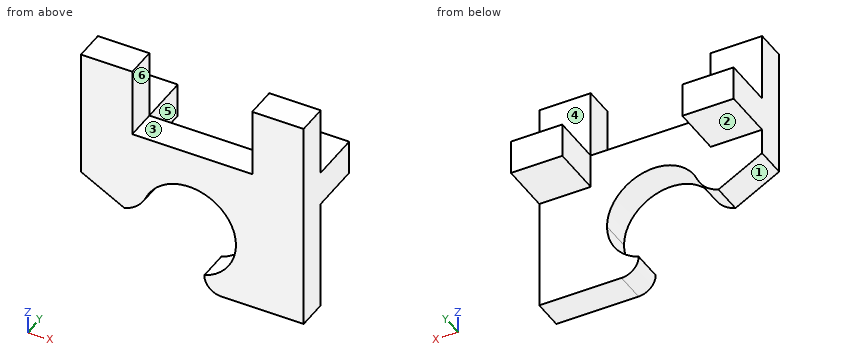
```python
from build123d import *

# Parameters (mm, degrees)
BOSS_EXTRUDE1_DEPTH = 1.8
FILLET1_R           = 2
FILLET3_R           = 1
SKETCH2_W           = 3
SKETCH2_H           = 2
BOSS_EXTRUDE2_DEPTH = 3


# Some blends are built 0.0001 mm under size
with BuildPart() as part:
    # Sketch1 → Boss-Extrude1 (new body)
    with BuildSketch(Plane(origin=(0, 0, 0), x_dir=(1, 0, 0), z_dir=(0, 1, 0))):
        with BuildLine():
            Line((6.5, 2.5), (6.5, 0))
            Line((6.5, 0), (6.5, -4))
            Line((6.5, -4), (3.5, -4))
            Line((3.5, -4), (3.5, 0))
            Line((3.5, 0), (-3.5, 0))
            Line((-3.5, 0), (-3.5, -4))
            Line((-3.5, -4), (-6.5, -4))
            Line((-6.5, -4), (-6.5, 0))
            Line((-6.5, 0), (-6.5, 2.5))
            Line((-6.5, 2.5), (-6.5, 3.5))
            Line((-6.5, 3.5), (-3.95, 4.9))
            Line((-3.95, 4.9), (-2.95, 4.9))
            ThreePointArc((-2.95, 4.9), (-0.2, 2.15), (2.55, 4.9))
            ThreePointArc((2.55, 4.9), (2.040256682, 6.494913791), (0.7, 7.498557292))
            Line((0.7, 7.498557292), (0.7, 8.498557292))
            Line((0.7, 8.498557292), (6.5, 8.498557292))
            Line((6.5, 8.498557292), (6.5, 4.9))
            Line((6.5, 4.9), (6.5, 2.5))
        make_face()
    extrude(amount=BOSS_EXTRUDE1_DEPTH)

    # Fillet1
    # the kernel refuses this fillet: 2 mm, written as the material it takes off along each edge
    with BuildSketch(Plane(origin=(-2.95, -2.821440468, -4.9), x_dir=(0.20519567041703107, 0, 0.9787209698591857), z_dir=(0, 1, 0))) as fillet1_piece_1:
        with BuildLine():
            CenterArc((1.538967528, -1.95744194), FILLET1_R, 101.840953646, 48.860489585)
            Line((-0.20519567, -0.97872097), (-0.240078934, -0.95914655))
            ThreePointArc((-0.240078934, -0.95914655), (-0.141746674, -0.481152658), (-0.039148839, 0.008207827))
            Line((-0.039148839, 0.008207827), (0.008207827, 0.039148839))
            ThreePointArc((0.008207827, 0.039148839), (0.564288094, -0.018517333), (1.12036836, 0.039148839))
            Line((1.12036836, 0.039148839), (1.128576187, 0))
        make_face()
    extrude(amount=7.442880936, mode=Mode.SUBTRACT)

    # Fillet3
    fillet3_edges = [part.edges().sort_by_distance(p)[0] for p in [
        (0.7, 0.9, -8.498557292),
    ]]
    fillet(fillet3_edges, radius=FILLET3_R - 0.0001)  # a hair under: the kernel refuses the full size

    # Sketch2 → Boss-Extrude2 (add)
    with BuildSketch(Plane.XZ):
        with Locations((5, -1)):
            Rectangle(SKETCH2_W, SKETCH2_H)
        with Locations((-5, -1)):
            Rectangle(SKETCH2_W, SKETCH2_H)
    extrude(amount=BOSS_EXTRUDE2_DEPTH)


with BuildPart() as body_2:
    # Mirror3: mirrored copy
    add(part.part.mirror(Plane(origin=(0, 0, 0), x_dir=(0, 0, 1), z_dir=(0, -1, 0))))


solid = body_2.part
```
The listing builds one solid part. Answer for the finished solid, in the listing's coordinates (mm). Face numbers are marked on the shaded views. A direction names the side the tool comes from. Give positions to 0.01 mm unless a question says otherwise; leave off trailing zeros. Loops run counter-clockwise (first coordinate to the right, second up) from the corner with the lowest first, then second, coordinate; pieces in that order, holes last. Notation, with made-up numbers: M -29,62 L 22,62 A20 ccw 22,67 Z; hole C 70,54.25 d3. An arc over 180 degrees is marked long. One line per item, written item: value.
1. For the marked faces 4, 5 and 6, determine the directions among +Z, -Z, +X, -X, +Y, -Y from which every point of the face is accessible in a straight line to the end or side of a thin tool.
Found:
face 4: +Z, +X, -X, +Y
face 5: +Z, -Z, +Y
face 6: +Z, +Y, -Y
2. Section D-D on x = -4.75 is taken. Determine the outline of the cut face in (y, z), plus the area to 3 significant figures.
Found:
outline: M -1.8,-4.46 L 0,-4.46 L 0,-2 L 3,-2 L 3,0 L 0,0 L 0,4 L -1.8,4 Z
area: 21.2 mm^2
3. Find the intervals of material crossed by probe 1 along Z at (x, y) = (-5.25, 1.6); probe 2 along Y at (x, z) = (2.5, -6.75); probe 3 along X at (y, z) = (-1.05, 1), in increasing order.
Found:
probe 1: -2 to 0
probe 2: -1.8 to 0
probe 3: -6.5 to -3.5, 3.5 to 6.5
4. Section B-B on z = -3.25 is taken. Determine the outline of the cut face in (x, y), plus the area to 3 significant figures.
Found:
outline: M -6.5,-1.8 L -2.4,-1.8 L -2.4,0 L -6.5,0 Z; M 2,-1.8 L 6.5,-1.8 L 6.5,0 L 2,0 Z
area: 15.5 mm^2
5. Section A-A on y = 1.9 is taken. Determine the outline of the cut face in (x, z), plus the area to 3 significant figures.
Found:
outline: M -6.5,-2 L -3.5,-2 L -3.5,0 L -6.5,0 Z; M 3.5,-2 L 6.5,-2 L 6.5,0 L 3.5,0 Z
area: 12.0 mm^2
6. For a pull along X with two mould halves and no side action, classify the marked faces 1, 2 and 3 as pulls with the +X half, pulls with the -X half, needs draft (parallel to the pull), parting line crosses it, or undercut.
Found:
face 1: pulls with the -X half
face 2: needs draft
face 3: undercut
7. Each of these flat-tipped pins is pushed along its axis until it touches: P1, Ø2, axis at y = 0.5, z = 1, coming from the +X side; P2, Ø3.5, axis at x = 5, z = 2, coming from the +Y side; P3, Ø2.5, axis at x = 0, z = -5.5, coming from the +Y side; P4, Ø0.9, axis at x = 1, y = -0.5, coming from the +Z side. Where does it stop, or does it pass through?
Found:
P1: x = 6.5
P2: y = 0
P3: through
P4: z = 0
